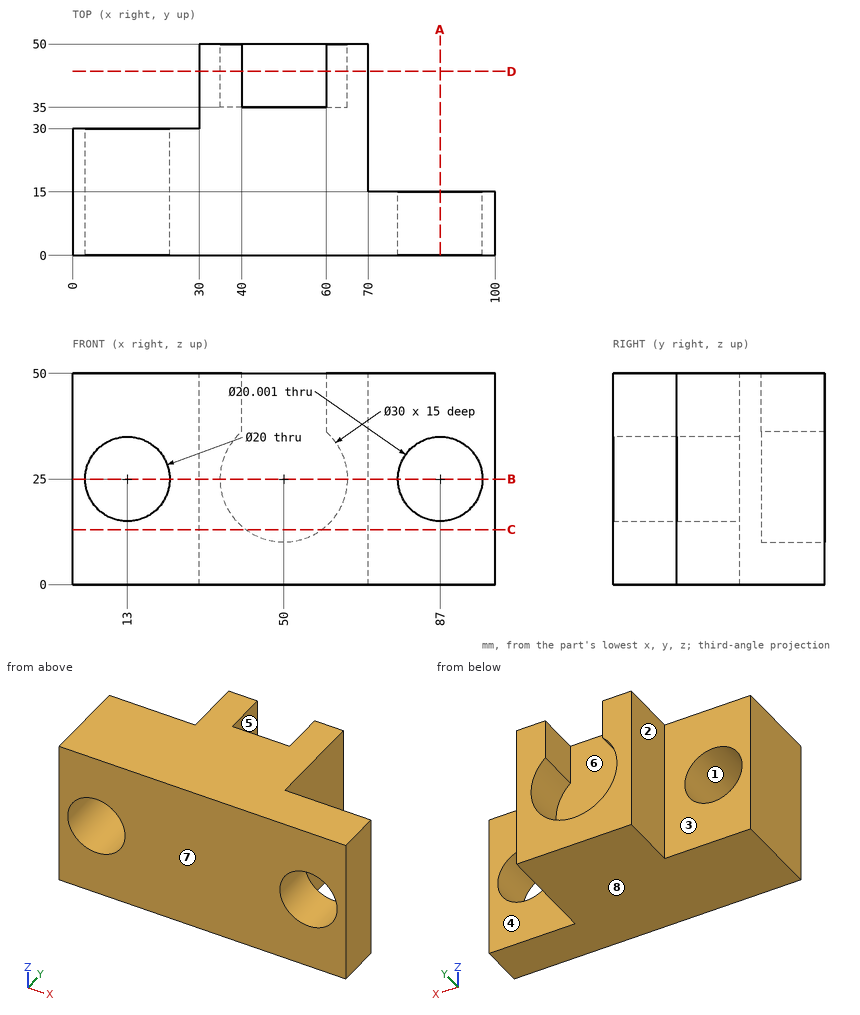
Could you check a few things on this drawing? It's one solid part, dimensions in mm from its lowest x, y, z. A direction names the side the tool comes from. Give positions to 0.01 mm unless a question says otherwise; leave off trailing zeros. Order: outer loops, then holes, each group sorted by start corner. A loop starts at its lowest first (then second) coordinate and runs counter-clockwise, first axis right, second up. Notation, with made-up numbers: (48.5, 11) - (76.5, 11) arc R22 cw to (76.5, 30) - close; hole circle Ø10 at (46.5, -4.75). An arc over 180 degrees is marked (long way). Answer as a JSON object with one key per item and string values. Group by question number.
Item 1: For P1, Ø12, axis at y = 37.5, z = 20.5, coming from the -X side; P2, Ø24, axis at x = 90.5, z = 17.5, coming from the +Y side; P3, Ø10.5, axis at y = 29.5, z = 27.5, coming from the +X side; P4, Ø16, axis at x = 13, z = 25, coming from the +Y side, each with a flat end and sliding along its axis, tell me the tip position at first contact or that it passes through.
Item 2: If we section it at C-C on z = 13: Please give me the cut outline in (x, y).
Item 3: Please list where these lines run through material, in increasing order: probe 1 along X at (y, z) = (14, 25); probe 2 along X at (y, z) = (40, 25); probe 3 along X at (y, z) = (7, 34).
Item 4: If we mould it in two halves opening along X, with no side actions, what happens to the marked faces 1, 2 and 3? For each: pulls with the +X half, pulls with the -X half, needs draft (parallel to the pull), parting line crosses it, or undercut.
Item 5: Which directions (+Z, -Z, +X, -X, +Y, -Y) give clear straight access to the entire face, cutting with the end or side of a thin tool? Please do the marked faces 4, 5, 6, 7 and 8.
Item 6: If we section it at D-D on y = 43.5: Please give me the cut outline in (x, z), and give its area (3 significant figures).
Item 7: If we section it at A-A on x = 87: Please give me the cut outline in (y, z), and give its area (3 significant figures).
Item 8: If we section it at B-B on z = 25: Please give me the cut outline in (x, y).
Result set:
{
 "1": {"P1": "x = 30", "P2": "y = 15", "P3": "x = 70", "P4": "through"},
 "2": {"outline": "(0, 0) - (100, 0) - (100, 15) - (70, 15) - (70, 50) - (59, 50) - (59, 35) - (41, 35) - (41, 50) - (30, 50) - (30, 30) - (0, 30) - close"},
 "3": {"probe 1": "0 to 3, 23 to 77, 97 to 100", "probe 2": "30 to 35, 65 to 70", "probe 3": "0 to 8.64, 17.36 to 82.64, 91.36 to 100"},
 "4": {"face 1": "undercut", "face 2": "pulls with the -X half", "face 3": "needs draft"},
 "5": {"face 4": "+Z, -Z, +X, +Y", "face 5": "+Z, +Y", "face 6": "+Y", "face 7": "+Z, -Z, +X, -X, -Y", "face 8": "-Z, +X, -X, +Y, -Y"},
 "6": {"outline": "(30, 0) - (70, 0) - (70, 50) - (60, 50) - (60, 36.18) arc R15 cw (long way) to (40, 36.18) - (40, 50) - (30, 50) - close", "area": "1,070 mm²"},
 "7": {"outline": "(0, 0) - (15, 0) - (15, 15) - (0, 15) - close; (0, 35) - (15, 35) - (15, 50) - (0, 50) - close", "area": "450 mm²"},
 "8": {"outline": "(0, 0) - (3, 0) - (3, 30) - (0, 30) - close; (23, 0) - (77, 0) - (77, 15) - (70, 15) - (70, 50) - (65, 50) - (65, 35) - (35, 35) - (35, 50) - (30, 50) - (30, 30) - (23, 30) - close; (97, 0) - (100, 0) - (100, 15) - (97, 15) - close"}
}
